```python
from build123d import *

# Parameters (mm, degrees)
F0_W     = 20
F0_H     = 20
F1_DEPTH = 20
F3_DEPTH = 20
F5_DEPTH = 20
F6_R     = 5
F7_DEPTH = 20


with BuildPart() as f1:
    # F0 (on Top) → F1 (new body)
    with BuildSketch(Plane.XY):
        with Locations((10, 10)):
            Rectangle(F0_W, F0_H)
    extrude(amount=F1_DEPTH)

    # F2 (on face) → F3 (cut)
    with BuildSketch(Plane.XY.offset(20)):
        with BuildLine():
            Line((4.0428322988, 9.9974628538), (15.9571677012, 9.9974628538))
            ThreePointArc((15.9571677012, 9.9974628538), (10, 15.954630555), (4.0428322988, 9.9974628538))
        make_face()
        with BuildLine():
            ThreePointArc((4.0428322988, 9.9974628538), (10, 4.0402951526), (15.9571677012, 9.9974628538))
            Line((15.9571677012, 9.9974628538), (4.0428322988, 9.9974628538))
        make_face()
    extrude(amount=-F3_DEPTH, mode=Mode.SUBTRACT)

    # F4 (on face) → F5 (cut)
    with BuildSketch(Plane(origin=(0, 20, 0), x_dir=(-1, 0, 0), z_dir=(0, 1, 0))):
        with BuildLine():
            Line((-15, 10), (-5, 10))
            ThreePointArc((-5, 10), (-10, 15), (-15, 10))
        make_face()
        with BuildLine():
            ThreePointArc((-15, 10), (-10, 5), (-5, 10))
            Line((-5, 10), (-15, 10))
        make_face()
    extrude(amount=-F5_DEPTH, mode=Mode.SUBTRACT)

    # F6 (on face) → F7 (cut)
    with BuildSketch(Plane.YZ.offset(20)):
        with Locations((10, 10)):
            Circle(F6_R)
    extrude(amount=-F7_DEPTH, mode=Mode.SUBTRACT)


solid = f1.part
```
Geometry check sheet. Reference: the model listing, model coordinates, mm. Coordinates: 2 decimals unless noted, no trailing zeros. Loops run counter-clockwise (first coordinate to the right, second up) from the corner with the lowest first, then second, coordinate; pieces in that order, holes last. Notation, with made-up numbers: (44, -33) - (72, -33) arc R33 cw to (72, -1) - close; hole circle Ø3 at (73.5, 16). An arc over 180 degrees is marked (long way). One line per item, written item: value. Start each with the question number.
(1) Cross-section at A-A on z = 10. Enter the section's corners in (x, y), plus the area to 3 significant figures.
(2) Cross-section at C-C on y = 2.75. Enter the section's corners in (x, z), plus the area to 3 significant figures.
(3) Cross-section at B-B on x = 10. Enter the section's corners in (y, z), plus the area to 3 significant figures.
(4) Depth check by flat-ended pin: P1, Ø6, axis at y = 10, z = 10, coming from the +X side; P2, Ø4, axis at x = 9, y = 15, coming from the +Z side. Enter the tip coordinate at first touch or a pass-through.
(5) Mould release check, pull along Y, two halves, no side actions. Record for faces 1 (the cylindrical face through (10.78, 4.09, 17.21)), 2 (the flat face through (8, 20, 5)), 3 (the flat face through (5, 15, 0)): released by +Y, released by -Y, zero draft, split by the parting line, or undercut.
(6) Material ranges on line 1 (Z direction, x = 10, y = 16.65); line 2 (X direction, y = 17.5, z = 10.25), recorded low to high. Write a range as [from, to].
Results below:
1. outline: (0, 0) - (5, 0) - (5, 5) - (0, 5) - close; (0, 15) - (5, 15) - (5, 20) - (0, 20) - close; (15, 0) - (20, 0) - (20, 5) - (15, 5) - close; (15, 15) - (20, 15) - (20, 20) - (15, 20) - close
1. area: 100 mm2
2. outline: (0, 0) - (20, 0) - (20, 20) - (0, 20) - close; hole circle Ø10 at (10, 10)
2. area: 321 mm2
3. outline: (0, 0) - (4.04, 0) - (4.04, 5) - (0, 5) - close; (0, 15) - (4.04, 15) - (4.04, 20) - (0, 20) - close; (15.95, 0) - (20, 0) - (20, 5) - (15.95, 5) - close; (15.95, 15) - (20, 15) - (20, 20) - (15.95, 20) - close
3. area: 80.9 mm2
4. P1: passes through
4. P2: stops at z = 20
5. face 1: undercut
5. face 2: released by +Y
5. face 3: zero draft
6. line 1: z = [0, 5], [15, 20]
6. line 2: x = [0, 5.01], [14.99, 20]
